from build123d import *

# Parameters (mm, degrees)
SKETCH1_R           = 1.6
SKETCH1_W           = 65
SKETCH1_H           = 65
BOSS_EXTRUDE1_DEPTH = 3
FILLET1_R           = 2
FILLET2_R           = 5


with BuildPart() as part:
    # Sketch1 → Boss-Extrude1 (new body)
    with BuildSketch(Plane(origin=(0, 0, 0), x_dir=(1, 0, 0), z_dir=(0, 1, 0))):
        Polygon((-50, 50), (-50, 41.75), (-40, 41.75), (-40, -22.5), (-50, -22.5), (-50, -50), (-41.5, -50), (-41.5, -30), (41.5, -30), (41.5, -50), (50, -50), (50, -23.25), (40, -23.25), (40, 42.5), (50, 42.5), (50, 50), align=None)
        with Locations((-45, -45)):
            Circle(SKETCH1_R, mode=Mode.SUBTRACT)
        with Locations((-35.75, -26.5)):
            Circle(SKETCH1_R, mode=Mode.SUBTRACT)
        with Locations((45, -45)):
            Circle(SKETCH1_R, mode=Mode.SUBTRACT)
        with Locations((35.75, -26.5)):
            Circle(SKETCH1_R, mode=Mode.SUBTRACT)
        with Locations((0, 9.25)):
            Rectangle(SKETCH1_W, SKETCH1_H, mode=Mode.SUBTRACT)
        with Locations((-45, 45)):
            Circle(SKETCH1_R, mode=Mode.SUBTRACT)
        with Locations((-35.75, 45)):
            Circle(SKETCH1_R, mode=Mode.SUBTRACT)
        with Locations((35.75, 45)):
            Circle(SKETCH1_R, mode=Mode.SUBTRACT)
        with Locations((45, 45)):
            Circle(SKETCH1_R, mode=Mode.SUBTRACT)
    extrude(amount=BOSS_EXTRUDE1_DEPTH)

    # Fillet1
    fillet1_edges = [part.edges().sort_by_distance(p)[0] for p in [
        (50, 1.5, 23.25),
        (41.5, 1.5, 50),
        (-41.5, 1.5, 50),
        (-50, 1.5, 22.5),
        (-50, 1.5, -41.75),
        (50, 1.5, -42.5),
    ]]
    fillet(fillet1_edges, radius=FILLET1_R)

    # Fillet2
    fillet2_edges = [part.edges().sort_by_distance(p)[0] for p in [
        (50, 1.5, 50),
        (-50, 1.5, 50),
        (-50, 1.5, -50),
        (50, 1.5, -50),
    ]]
    fillet(fillet2_edges, radius=FILLET2_R)


solid = part.part
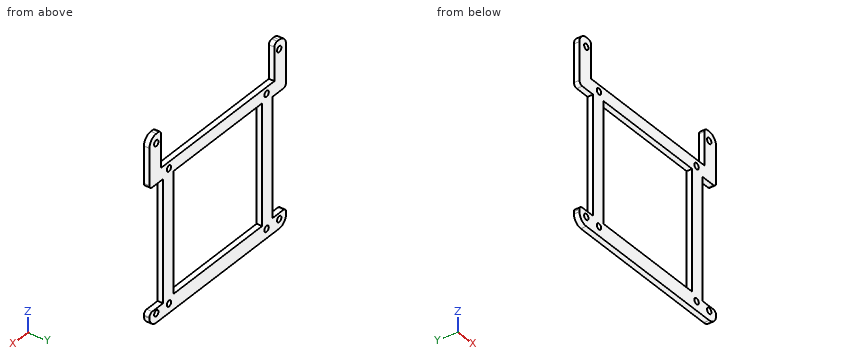
Build history of the part. All positions in model axes, mm. Give positions to 0.01 mm unless a question says otherwise; leave off trailing zeros. Order: outer loops, then holes, each group sorted by start corner. A loop starts at its lowest first (then second) coordinate and runs counter-clockwise, first axis right, second up. Notation, with made-up numbers: M 10,9.25 L 22,9.25 A25 cw 22,25.25 Z; hole C -10,-14.5 d7. An arc over 180 degrees is marked long. Put each result on its own line as item: value.
Item 1: Wall check: probe 1 along Z at (x, y) = (-45, 1.35); probe 2 along Z at (x, y) = (-35.75, 0.8); probe 3 along X at (y, z) = (1.1, -45). Give the ranges that are in metal, low to high.
Results are:
probe 1: -50 to -46.6, -43.4 to -41.75, 22.5 to 43.4, 46.6 to 50
probe 2: -50 to -46.6, -43.4 to 24.9, 28.1 to 30
probe 3: -50 to -46.6, -43.4 to -37.35, -34.15 to 34.15, 37.35 to 43.4, 46.6 to 50
Item 2: Cut at C-C on x = 35.75. Write the cut outline in (y, z).
Results are:
outline: M 0,-50 L 3,-50 L 3,-46.6 L 0,-46.6 Z; M 0,-43.4 L 3,-43.4 L 3,24.9 L 0,24.9 Z; M 0,28.1 L 3,28.1 L 3,30 L 0,30 Z
Item 3: Cut at A-A on z = 21. Write the cut outline in (x, y).
Results are:
outline: M -40,0 L -32.5,0 L -32.5,3 L -40,3 Z; M 32.5,0 L 40,0 L 40,3 L 32.5,3 Z
Item 4: Cut at D-D on y = 0.85. Count the separate pieces of the cut face and the enclosed holes in it, then the cut area to 3 significant figures.
Results are:
separate pieces: 1
enclosed holes: 9
area: 2,720 mm2
Item 5: Cut at B-B on x = -4. Write the cut outline in (y, z).
Results are:
outline: M 0,-50 L 3,-50 L 3,-41.75 L 0,-41.75 Z; M 0,23.25 L 3,23.25 L 3,30 L 0,30 Z
Item 6: Drop flat-ended pins along their axis: pin 1 Ø5 at (x, z) = (35.75, 26.5) entering from -Y; pin 2 Ø1.5 at (y, z) = (2, -18.5) entering from +X; pin 3 Ø0.9 at (x, y) = (17.5, 2) entering from +Z; pin 4 Ø1.5 at (y, z) = (1, -5.5) entering from -X. Give the stop position or say it passes through.
Results are:
pin 1: y = 0
pin 2: x = 40
pin 3: z = 30
pin 4: x = -40
